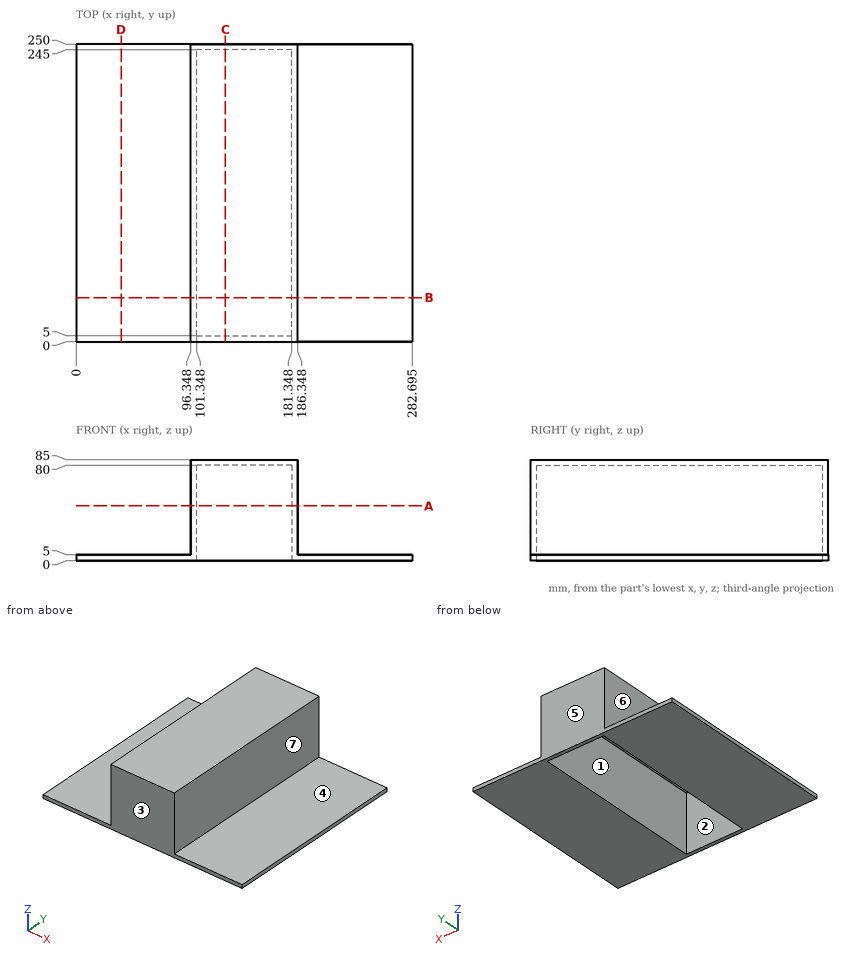
Input: dimensioned drawing with shaded views. Units: mm. Origin: part minimum x, y, z. A direction names the side the tool comes from. Round coordinates to 2 decimals unless told otherwise and drop trailing zeros. Order: outer loops, then holes, each group sorted by start corner. A loop starts at its lowest first (then second) coordinate and runs counter-clockwise, first axis right, second up.
Q1. Section C-C, the plane x = 125.5. Output: boundary loops of the cut face in (y, z).
Result sheet:
outline: (0, 0) - (5, 0) - (5, 80) - (245, 80) - (245, 0) - (250, 0) - (250, 85) - (0, 85) - close
Q2. Pin query (flat end, axial travel): pin 1 (24 mm diameter, centred on y = 65.5, z = 37.5, fed in from -X); pin 2 (5 mm diameter, centred on y = 81, z = 56.5, fed in from +X). Return the tip coordinate at first contact, or that it passes through.
Result sheet:
pin 1: stops at x = 96.35
pin 2: stops at x = 186.35
Q3. Access query for the marked faces 5, 6 and 7. Directions: +Z, -Z, +X, -X, +Y, -Y. A direction counts if a zero-diameter tool reaches every point of the face in a straight line with its end or side. Return the directions, or none.
Result sheet:
face 5: +Z, -Z, +X, -X, +Y
face 6: +Z, -X, +Y, -Y
face 7: +Z, +X, +Y, -Y
Q4. Material intervals for probe 1 along Y at (x, z) = (167, 15); probe 2 along X at (y, z) = (211.5, 72); probe 3 along Z at (x, y) = (84.5, 54), sorted ascending.
Result sheet:
probe 1: y = 0 to 5, 245 to 250
probe 2: x = 96.35 to 101.35, 181.35 to 186.35
probe 3: z = 0 to 5
Q5. Section A-A, the plane z = 46. Output: boundary loops of the cut face in (x, y), and give its area (3 significant figures).
Result sheet:
outline: (96.35, 0) - (186.35, 0) - (186.35, 250) - (96.35, 250) - close; hole (101.35, 5) - (181.35, 5) - (181.35, 245) - (101.35, 245) - close
area: 3,300 mm2
Q6. Mould query, pull axis Y, two halves, no side actions, for the marked faces 1, 2, 3 and 4. Classes: released by +Y, released by -Y, zero draft, split by the parting line, or undercut.
Result sheet:
face 1: undercut
face 2: undercut
face 3: released by -Y
face 4: zero draft
Q7. Section B-B, the plane y = 37. Output: boundary loops of the cut face in (x, z) (1 decimal), and give its area (3 significant figures).
Result sheet:
outline: (0, 0) - (101.3, 0) - (101.3, 80) - (181.3, 80) - (181.3, 0) - (282.7, 0) - (282.7, 5) - (186.3, 5) - (186.3, 85) - (96.3, 85) - (96.3, 5) - (0, 5) - close
area: 2,210 mm2
Q8. Section D-D, the plane x = 38. Output: boundary loops of the cut face in (y, z).
Result sheet:
outline: (0, 0) - (250, 0) - (250, 5) - (0, 5) - close
